Autodesk Inventor part; units mm, degrees
ref_plane "YZ Plane" through (0, 0, 0) normal (1, 0, 0) x (0, 1, 0)
ref_plane "XZ Plane" through (0, 0, 0) normal (0, 1, 0) x (-1, 0, 0)
ref_plane "XY Plane" through (0, 0, 0) normal (0, 0, 1) x (1, 0, 0)
sketch "Sketch1" plane through (0, 0, 0) normal (0, 1, 0) x (-1, 0, 0)
  line L0 (-75, 114) -> (75, 114)
  line L1 (75, 114) -> (75, -114)
  line L2 (75, -114) -> (-75, -114)
  line L3 (-75, -114) -> (-75, 114)
  line L4 (-75, 114) -> (75, -114) construction
  line L5 (75, 114) -> (-75, -114) construction
  line L6 (75.8, 114.8) -> (-75.8, 114.8)
  line L7 (-75.8, 114.8) -> (-75.8, -114.8)
  line L8 (-75.8, -114.8) -> (75.8, -114.8)
  line L9 (75.8, -114.8) -> (75.8, 114.8)
  point P0 (0, 0)
  dimension "d0" = 150
  dimension "d1" = 228
  dimension "d2" = 0.8
extrude "Extrusion1" add sketch "Sketch1" along normal blind 101.6
sketch "Sketch3" plane through (0, 0, 0) normal (0, -1, 0) x (1, 0, 0)
  line L0 (75.8, 114.8) -> (75.8, -114.8)
  line L1 (75.8, -114.8) -> (-75.8, -114.8)
  line L2 (75.8, 114.8) -> (75.8, -114.8)
  line L3 (75.8, -114.8) -> (90.8, -114.8)
  line L4 (90.8, -114.8) -> (90.8, 114.8)
  line L5 (90.8, 114.8) -> (75.8, 114.8)
  line L6 (75.8, -114.8) -> (-75.8, -114.8)
  line L7 (-75.8, -114.8) -> (-75.8, -129.8)
  line L8 (-75.8, -129.8) -> (75.8, -129.8)
  line L9 (75.8, -129.8) -> (75.8, -114.8)
  line L10 (-75.8, 114.8) -> (75.8, 114.8)
  line L11 (-75.8, -114.8) -> (-75.8, 114.8)
  line L12 (-75.8, 114.8) -> (-90.8, 114.8)
  line L13 (-90.8, 114.8) -> (-90.8, -114.8)
  line L14 (-90.8, -114.8) -> (-75.8, -114.8)
  line L15 (-75.8, 114.8) -> (75.8, 114.8)
  line L16 (75.8, 114.8) -> (75.8, 129.8)
  line L17 (75.8, 129.8) -> (-75.8, 129.8)
  line L18 (-75.8, 129.8) -> (-75.8, 114.8)
  point P0 (0, 0)
  dimension "d11" = 15
  dimension "d12" = 15
  dimension "d13" = 15
  dimension "d14" = 15
extrude "Extrusion3" add sketch "Sketch3" against normal blind 0.8 contours L5 L4 L3 L0 | L10 L18 L17 L16 | L9 L8 L7 L1 | L11 L14 L13 L12
fillet "Fillet1" radius 2 4 edges at (75, 0, 0) (0, 0, -114) (-75, 0, 0) (0, 0, 114)
sketch "Sketch4" plane through (0, 0.8, 0) normal (0, 1, 0) x (1, 0, 0)
  line L0 (82.25, 120.65) -> (-82.25, 120.65) construction
  line L1 (-82.25, 120.65) -> (-82.25, -120.65) construction
  line L2 (-82.25, -120.65) -> (82.25, -120.65) construction
  line L3 (82.25, -120.65) -> (82.25, 120.65) construction
  line L4 (82.25, 120.65) -> (-82.25, -120.65) construction
  line L5 (-82.25, 120.65) -> (82.25, -120.65) construction
  line L6 (0, 0) -> (0, -60) construction
  line L7 (0, 0) -> (60, 0) construction
  point P0 (44.45, 120.65)
  point P1 (-44.45, 120.65)
  point P2 (-82.25, 88.9)
  point P3 (-82.25, 0)
  point P4 (-82.25, -88.9)
  point P5 (-44.45, -120.65)
  point P6 (44.45, -120.65)
  point P7 (82.25, -88.9)
  point P8 (82.25, 0)
  point P9 (82.25, 88.9)
  dimension "d18" = 164.5
  dimension "d19" = 241.3
  dimension "d20" = 88.9
  dimension "d21" = 60
  dimension "d22" = 90
  dimension "d23" = 88.9
  dimension "d24" = 88.9
hole "Hole1" at (44.45, 0.8, -120.65) at (-44.45, 0.8, -120.65) at (-82.25, 0.8, -88.9) at (-82.25, 0.8, 0) at (-82.25, 0.8, 88.9) at (-44.45, 0.8, 120.65) at (44.45, 0.8, 120.65) at (82.25, 0.8, 88.9) at (82.25, 0.8, 0) at (82.25, 0.8, -88.9) direction (0, -1, 0) diameter 4.496 end through all
sketch "Sketch8" plane through (75.8, 101.6, 114.8) normal (1, 0, 0) x (0, 0, -1)
  line L0 (0.8, -99.6) -> (0.8, 0)
  line L1 (0.8, 0) -> (229, 0)
  line L2 (229, 0) -> (229, -25.4)
  line L3 (229, -25.4) -> (0.8, -25.4)
  line L4 (0.8, -25.4) -> (0.8, 0)
  point P0 (114.8, -101.6)
  dimension "d48" = 25.4
extrude "Extrusion7" cut sketch "Sketch8" against normal through all
sketch "Sketch9" plane through (75.8, 0.8, 114.8) normal (1, 0, 0) x (0, 0, -1)
  line L0 (0, 100.8) -> (14.1421, 114.9421)
  line L1 (0, 100.8) -> (20, 100.8) construction
  line L2 (14.5421, 114.5421) -> (0.8, 100.8)
  line L3 (14.1421, 114.9421) -> (14.5421, 114.5421)
  line L4 (229.6, 0) -> (229.6, 100.8)
  line L5 (229.6, 100.8) -> (215.4579, 114.9421)
  line L6 (229.6, 100.8) -> (249.6, 100.8) construction
  line L7 (215.1579, 114.6421) -> (229, 100.8)
  line L8 (229, 100.8) -> (229.6, 100.8)
  line L9 (229, 100.8) -> (229.6, 100.8)
  line L10 (215.4579, 114.9421) -> (215.1579, 114.6421)
  line L11 (0.8, 100.8) -> (0, 100.8)
  line L12 (0, 100.8) -> (0.8, 100.8)
  point P0 (114.8, -0.8)
  dimension "d51" = 20
  dimension "d52" = 45
  dimension "d53" = 20
  dimension "d54" = 135
extrude "Extrusion8" add sketch "Sketch9" against normal up to surface (151.6 mm away)
sketch "Sketch10" plane through (0, 0.8, 0) normal (0, 1, 0) x (1, 0, 0)
  line L0 (75.8, 114.2) -> (75.8, -114)
  line L1 (-75.8, -114) -> (-75.8, 114.2)
  line L2 (-75.8, -114.8) -> (75.8, -114.8)
  line L3 (75.8, 114.8) -> (-75.8, 114.8)
  line L4 (90.8, -114.8) -> (90.8, 114.8)
  line L5 (90.8, -54.8) -> (75.8, -54.8)
  line L6 (75.8, -54.8) -> (75.8, 54.8)
  line L7 (75.8, 54.8) -> (90.8, 54.8)
  line L8 (90.8, 54.8) -> (90.8, -54.8)
  line L9 (90.8, 114.8) -> (75.8, 114.8)
  line L10 (75.8, -114.8) -> (90.8, -114.8)
  line L11 (0, 0) -> (0, 22) construction
  line L12 (-90.8, -54.8) -> (-75.8, -54.8)
  line L13 (-75.8, -54.8) -> (-75.8, 54.8)
  line L14 (-75.8, 54.8) -> (-90.8, 54.8)
  line L15 (-90.8, 54.8) -> (-90.8, -54.8)
  dimension "d57" = 60
  dimension "d58" = 60
extrude "Extrusion9" cut sketch "Sketch10" against normal through all
properties part number "chimneyHousing"
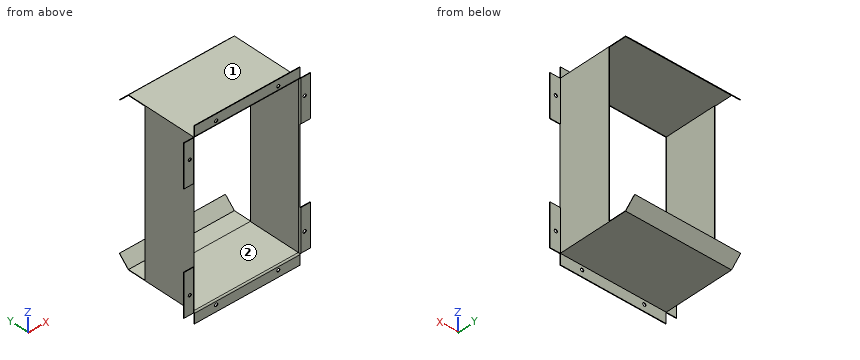
Can you work these out from the model? Positions are in its coordinate system, mm. Face numbers are marked on the shaded views. A direction names the side the tool comes from. Coordinates: 2 decimals unless noted, no trailing zeros. Order: outer loops, then holes, each group sorted by start corner. A loop starts at its lowest first (then second) coordinate and runs counter-clockwise, first axis right, second up. Notation, with made-up numbers: (-7, -8.75) - (16, -8.75) arc R25 cw to (16, 26.25) - close; hole circle Ø1 at (28.5, -30.75). An arc over 180 degrees is marked (long way). Answer in a Markdown table with one row per item.
1. If I drill on line 1 along Z through (x, y) = (59, 7); line 2 along X through (y, z) = (56.5, -96); line 3 along Z through (x, y) = (-9, 97), over which ranges is the centre line in solid material (lowest first)?
Reply:
| item | result |
|---|---|
| line 1 | z = -114.8 to -114, 114 to 114.8 |
| line 2 | x = -75.8 to -75, 75 to 75.8 |
| line 3 | z = -114.8 to -114.2, 114 to 114.8 |
2. Suppose I cut it at B-B (x = 24.5). Please give me the cut outline in (y, z).
Reply:
| item | result |
|---|---|
| outline | (0, -129.8) - (0.8, -129.8) - (0.8, -114.8) - (101.6, -114.8) - (115.74, -100.66) - (115.44, -100.36) - (101.6, -114.2) - (76.2, -114.2) - (76.2, -114) - (2, -114) arc R2 ccw to (0, -116) - close; (0, 116) arc R2 ccw to (2, 114) - (101.6, 114) - (115.34, 100.26) - (115.74, 100.66) - (101.6, 114.8) - (0.8, 114.8) - (0.8, 129.8) - (0, 129.8) - close |
3. Suppose I cut it at A-A (y = 21). Please give me the cut outline in (x, z).
Reply:
| item | result |
|---|---|
| outline | (-75.8, -114.8) - (75.8, -114.8) - (75.8, 114.8) - (-75.8, 114.8) - close; hole (-75, -114) - (75, -114) - (75, 114) - (-75, 114) - close |
4. For pin 1 (0.6 mm diameter, centred on x = -85.5, y = 0, fed in from +Z); pin 2 (6 mm diameter, centred on x = 14.5, y = 41.5, fed in from -Z); pin 3 (7.5 mm diameter, centred on x = 81.5, z = -74, fed in from +Y); pin 4 (2.5 mm diameter, centred on x = 82.25, z = -88.9, fed in from +Y), each with a flat end and sliding along its axis, tell me the tip position at first contact or that it passes through.
Reply:
| item | result |
|---|---|
| pin 1 | stops at z = 114.8 |
| pin 2 | stops at z = -114.8 |
| pin 3 | stops at y = 0.8 |
| pin 4 | passes through |
5. Suppose I cut it at C-C (z = 75.5). Please give me the cut outline in (x, y).
Reply:
| item | result |
|---|---|
| outline | (-90.8, 0) - (-77, 0) arc R2 ccw to (-75, 2) - (-75, 76.2) - (-75.8, 76.2) - (-75.8, 0.8) - (-90.8, 0.8) - close; (75, 2) arc R2 ccw to (77, 0) - (90.8, 0) - (90.8, 0.8) - (75.8, 0.8) - (75.8, 76.2) - (75, 76.2) - close |
6. For the marked faces 1 and 2, which set-ups out of +Z, -Z, +X, -X, +Y, -Y let a thin tool reach every point of the face, with its end or its side?
Reply:
| item | result |
|---|---|
| face 1 | +Z, +X, -X, +Y |
| face 2 | -Y |
7. Suppose I cut it at D-D (y = 82). Please give me the cut outline in (x, z), and give its area (3 significant figures).
Reply:
| item | result |
|---|---|
| outline | (-75.8, -114.8) - (75.8, -114.8) - (75.8, -114.2) - (-75.8, -114.2) - close; (-75.8, 114) - (75.8, 114) - (75.8, 114.8) - (-75.8, 114.8) - close |
| area | 212 mm^2 |
